Design review of the part built by this model. Coordinates are the model's own, in mm. A direction names the side the tool comes from. Round coordinates to 2 decimals unless told otherwise and drop trailing zeros. Order: outer loops, then holes, each group sorted by start corner. A loop starts at its lowest first (then second) coordinate and runs counter-clockwise, first axis right, second up. Notation, with made-up numbers: M 10,59.25 L 24,59.25 A24 ccw 24,72.25 Z; hole C 67,30 d7. An arc over 180 degrees is marked long. Write each question's results on one line, items separated by ' | '. Start each with the question number.
Item 1: Take a section at C-C, the plane x = 139. Write out the cut boundary in (y, z), plus the area to 3 significant figures.
Item 2: Take a section at D-D, the plane y = 188. Write out the cut boundary in (x, z), plus the area to 3 significant figures.
Item 3: The part is to be moulded in two halves that separate along Y. For faces 5 (the flat face through (705.1, 1928.9, -57.6)), 6 (the cylindrical face through (726.22, 1640.99, 57.39)), 7 (the flat face through (1, 362, -62.5)), say which applies: +Y half, -Y half, draft (parallel to the pull), parting line (faces both ways), or undercut.
Item 4: Take a section at B-B, the plane y = 852. Write out the cut boundary in (x, z), plus the area to 3 significant figures.
Item 5: Clearance check with flat-ended pins moving along their axes: pin 1 (10 mm diameter, centred on y = 1132, z = -88, fed in from +X); pin 2 (8 mm diameter, centred on y = 1630.5, z = -26, fed in from +X); pin 3 (5 mm diameter, centred on y = 1611, z = -1, fed in from -X). State where each tip first meets the part, or that it passes through.
Item 6: Wall thickness on line 1 (Z direction, x = 323.5, y = 1283); line 2 (X direction, y = 1594, z = -71.5); line 3 (Z direction, x = 531, y = 1920): over which ranges is each line inside the solid? List them lowest first. Write a range as [from, to].
Item 7: Take a section at A-A, the plane x = 0. Write out the cut boundary in (y, z).
Item 8: Machinability: for faces 1 (the flat face through (660.81, 1857.21, -77.32)), 2 (the flat face through (317, 1094, -89)), 3 (the flat face through (730, 1663, 65)), 4 (the flat face through (660.81, 1857.21, 0.7)), which of the approach directions +Z, -Z, +X, -X, +Y, -Y give a long, thin tool a straight path to every point of the face, cutting with its end or side? Answer none if there is none.
```python
from build123d import *

# Parameters (mm, degrees)
BOSS_EXTRUDE7_DEPTH     = 132.5
SKETCH1_4_R             = 60
BOSS_EXTRUDE8_DEPTH     = 107.5
BOSS_EXTRUDE11_DEPTH    = 90
BOSS_EXTRUDE13_START    = 15
BOSS_EXTRUDE13_DEPTH    = 15
BOSS_EXTRUDE14_DEPTH    = 15
CUT_EXTRUDE1_DEPTH      = 2219.375045612
CUT_EXTRUDE1_DEPTH_BACK = 2219.375045612
SKETCH9_R               = 25
CUT_EXTRUDE2_DEPTH      = 2219.375045612
CUT_EXTRUDE2_DEPTH_BACK = 2219.375045612
SKETCH10_R              = 25
SKETCH10_R_2            = 30
CUT_EXTRUDE4_DEPTH      = 89
BOSS_EXTRUDE16_DEPTH    = 7.5
LPATTERN1_COUNT         = 2
LPATTERN1_PITCH         = 70
LPATTERN1_COL_COUNT     = 2
LPATTERN1_COL_PITCH     = 70


with BuildPart() as part:
    # Sketch1 → Boss-Extrude7 (new, symmetric)
    with BuildSketch(Plane.XY):
        with BuildLine():
            ThreePointArc((-60, 0), (0, -60), (60, 0))
            ThreePointArc((60, 0), (10.41889066, 59.088465181), (-56.381557247, 20.5212086))
            Line((-56.381557247, 20.5212086), (-60, 0))
        make_face()
    extrude(amount=BOSS_EXTRUDE7_DEPTH, both=True)



with BuildPart() as body_2:
    # Sketch1_4 → Boss-Extrude8 (new, symmetric)
    with BuildSketch(Plane.XY):
        with Locations((281.31004782, 1595.38855988)):
            Circle(SKETCH1_4_R)
    extrude(amount=BOSS_EXTRUDE8_DEPTH, both=True)


with BuildPart() as part_1:
    add(part.part)

    add(body_2.part)  # Boss-Extrude11 merges body 2
    # Sketch1_7 → Boss-Extrude11 (add, symmetric)
    with BuildSketch(Plane.XY):
        with BuildLine():
            ThreePointArc((-56.381557247, 20.5212086), (10.41889066, 59.088465181), (60, 0))
            Line((60, 0), (646.722444698, 1569.08117349))
            Line((646.722444698, 1569.08117349), (742.972852685, 1826.485171715))
            Line((742.972852685, 1826.485171715), (576.320357346, 1888.801106118))
            ThreePointArc((576.320357346, 1888.801106118), (530.902858358, 1891.953630178), (491.119863482, 1869.817665301))
            Line((491.119863482, 1869.817665301), (436.375853911, 1813.868381125))
            Line((436.375853911, 1813.868381125), (281.31004782, 1655.38855988))
            ThreePointArc((281.31004782, 1655.38855988), (323.736454692, 1637.814966751), (341.31004782, 1595.38855988))
            ThreePointArc((341.31004782, 1595.38855988), (281.31004782, 1535.38855988), (221.31004782, 1595.38855988))
            Line((221.31004782, 1595.38855988), (-56.381557247, 20.5212086))
        make_face()
    extrude(amount=BOSS_EXTRUDE11_DEPTH, both=True)

    # Sketch7 → Boss-Extrude13 (add)
    with BuildSketch(Plane.XY.offset(50).offset(BOSS_EXTRUDE13_START)):
        with BuildLine():
            Line((491.119863482, 1869.817665301), (436.375853911, 1813.868381125))
            Line((436.375853911, 1813.868381125), (560.751749188, 2047.345886438))
            ThreePointArc((560.751749188, 2047.345886438), (620.317436407, 2071.284752328), (668.241381159, 2028.571336245))
            Line((668.241381159, 2028.571336245), (742.972852685, 1826.485171715))
            Line((742.972852685, 1826.485171715), (576.320357346, 1888.801106118))
            ThreePointArc((576.320357346, 1888.801106118), (530.902858358, 1891.953630178), (491.119863482, 1869.817665301))
        make_face()
    boss_extrude13 = extrude(amount=-BOSS_EXTRUDE13_DEPTH)

    # Mirror1: Boss-Extrude13 across plane
    add(boss_extrude13.mirror(Plane.XY))

    # Sketch8 → Boss-Extrude14 (add)
    with BuildSketch(Plane.XY.offset(50)):
        with BuildLine():
            Line((710.056223746, 1557.555052999), (646.722444698, 1569.08117349))
            Line((646.722444698, 1569.08117349), (742.972852685, 1826.485171715))
            Line((742.972852685, 1826.485171715), (780.294600873, 1624.350387969))
            ThreePointArc((780.294600873, 1624.350387969), (762.1465459, 1573.106790346), (710.056223746, 1557.555052999))
        make_face()
    boss_extrude14 = extrude(amount=BOSS_EXTRUDE14_DEPTH)

    # Mirror2: Boss-Extrude14 across plane
    add(boss_extrude14.mirror(Plane.XY))

    # Sketch9 → Cut-Extrude1 (cut, two sides: drawn at the far end of the back side and taken through both)
    with BuildSketch(Plane.XY.offset(-CUT_EXTRUDE1_DEPTH_BACK)):
        with Locations((68.388115759, 250.844704195)):
            Circle(SKETCH9_R)
    extrude(amount=CUT_EXTRUDE1_DEPTH + CUT_EXTRUDE1_DEPTH_BACK, mode=Mode.SUBTRACT)

    # Sketch10 → Cut-Extrude2 (cut, two sides: drawn at the far end of the back side and taken through both)
    with BuildSketch(Plane.XY.offset(-CUT_EXTRUDE2_DEPTH_BACK)):
        Circle(SKETCH10_R)
        with Locations((281.31004782, 1595.38855988)):
            Circle(SKETCH10_R_2)
        with Locations(Location((609.837606949, 2011.284752328, 0), (0, 0, 180))):
            Circle(SKETCH10_R_2)
        with Locations(Location((720.799173277, 1616.585460717, 0), (0, 0, 180))):
            Circle(SKETCH10_R)
    extrude(amount=CUT_EXTRUDE2_DEPTH + CUT_EXTRUDE2_DEPTH_BACK, mode=Mode.SUBTRACT)

    # Sketch11 → Cut-Extrude4 (cut, symmetric)
    with BuildSketch(Plane.XY):
        with BuildLine():
            Line((-42.351656293, 42.501025978), (226.976301927, 1569.935778948))
            ThreePointArc((226.976301927, 1569.935778948), (328.238074608, 1558.001927218), (293.977396944, 1654.036136694))
            Line((293.977396944, 1654.036136694), (500.241290249, 1864.841250757))
            ThreePointArc((500.241290249, 1864.841250757), (533.065252826, 1882.248483551), (570.174440959, 1880.4229894))
            Line((570.174440959, 1880.4229894), (730.103837176, 1820.621005976))
            Line((730.103837176, 1820.621005976), (56.681618874, 19.677247823))
            ThreePointArc((56.681618874, 19.677247823), (13.474723345, 58.467356968), (-42.351656293, 42.501025978))
        make_face()
    extrude(amount=CUT_EXTRUDE4_DEPTH, both=True, mode=Mode.SUBTRACT)

    # Sketch13 → Boss-Extrude16 (add, symmetric)
    with BuildSketch(Plane.XY):
        with BuildLine():
            Line((-52.815446615, 40.745626997), (-57.605998913, 62.429992466))
            ThreePointArc((-57.605998913, 62.429992466), (-58.072295212, 66.315467027), (-57.773050391, 70.21736366))
            Line((-57.773050391, 70.21736366), (44.51864625, 650.342403118))
            ThreePointArc((44.51864625, 650.342403118), (45.368489936, 653.563955799), (46.741348728, 656.599725011))
            Line((46.741348728, 656.599725011), (59.96272179, 680.342403118))
            Line((59.96272179, 680.342403118), (-52.815446615, 40.745626997))
        make_face()
    boss_extrude16 = extrude(amount=BOSS_EXTRUDE16_DEPTH, both=True)

    # LPattern1: Boss-Extrude16 ×2
    with Locations(*[(0, 0, i * LPATTERN1_PITCH) for i in range(1, LPATTERN1_COUNT)]):
        add(boss_extrude16)

    # LPattern1 col: Boss-Extrude16 ×2
    with Locations(*[(0, 0, -i * LPATTERN1_COL_PITCH) for i in range(1, LPATTERN1_COL_COUNT)]):
        add(boss_extrude16)


solid = part_1.part
```
Results list:
1) outline: M 211.27,-90 L 1128.59,-90 L 1128.59,90 L 211.27,90 Z; hole M 239.82,-89 L 1071,-89 L 1071,89 L 239.82,89 Z | area: 17,200 mm²
2) outline: M -37,-77.5 L -26.85,-77.5 L -26.85,-90 L 130.3,-90 L 130.3,90 L -26.85,90 L -26.85,77.5 L -37,77.5 L -37,62.5 L -26.85,62.5 L -26.85,7.5 L -37,7.5 L -37,-7.5 L -26.85,-7.5 L -26.85,-62.5 L -37,-62.5 Z; hole M -16.7,-89 L 119.62,-89 L 119.62,89 L -16.7,89 Z | area: 4,480 mm²
3) face 5: +Y half | face 6: undercut | face 7: draft
4) outline: M 90.23,-90 L 378.59,-90 L 378.59,90 L 90.23,90 Z; hole M 100.38,-89 L 367.91,-89 L 367.91,89 L 100.38,89 Z | area: 4,280 mm²
5) pin 1: x = 485.16 | pin 2: x = 671.18 | pin 3: x = 222.76
6) line 1: [-90, -89], [89, 90] | line 2: [221.07, 251.34], [311.28, 341.29], [645.36, 656.04] | line 3: [-65, -50], [50, 65]
7) outline: M -60,-132.5 L -25,-132.5 L -25,132.5 L -60,132.5 Z; M 25,-132.5 L 60,-132.5 L 60,-90 L 340.28,-90 L 340.28,-77.5 L 397.86,-77.5 L 397.86,-62.5 L 340.28,-62.5 L 340.28,-7.5 L 397.86,-7.5 L 397.86,7.5 L 340.28,7.5 L 340.28,62.5 L 397.86,62.5 L 397.86,77.5 L 340.28,77.5 L 340.28,90 L 60,90 L 60,132.5 L 25,132.5 Z; hole M 60,-89 L 282.69,-89 L 282.69,89 L 60,89 Z
8) face 1: -Z, +X, +Y | face 2: none | face 3: +Z, +X, -Y | face 4: +X, +Y
